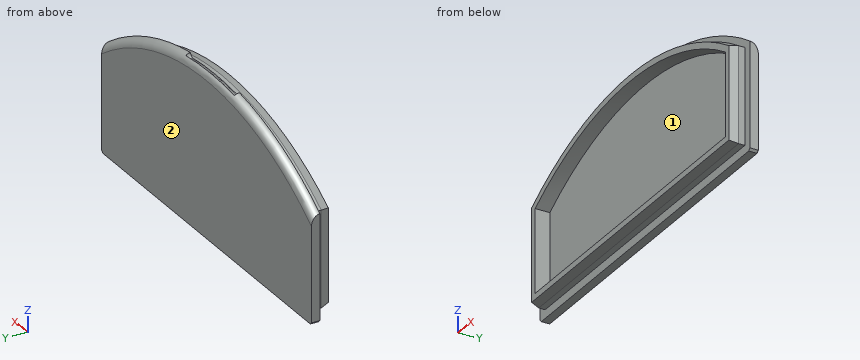
```python
from build123d import *
from OCP.BRepFilletAPI import BRepFilletAPI_MakeChamfer

# Parameters (mm, degrees)
EXTRUDE_1_DEPTH     = 4
CHAMFER_1_SIZE      = 1
EXTRUDE_2_DEPTH     = 7
CHAMFER_2_SIZE      = 4
CHAMFER_2_SIZE2     = 1.07179677
CUT_EXTRUDE_1_DEPTH = 2.5
FILLET_1_R          = 2
FILLET_2_R          = 4


with BuildPart() as part:
    # 스케치1 → 보스-돌출1 (new body)
    with BuildSketch(Plane(origin=(0, 0, 0), x_dir=(1, 0, 0), z_dir=(0, 1, 0))):
        with BuildLine():
            Line((85.8, -72), (85.8, -123.038042897))
            ThreePointArc((85.8, -123.038042897), (0, -150), (-85.8, -123.038042897))
            Line((-85.8, -123.038042897), (-85.8, -72))
            Line((-85.8, -72), (85.8, -72))
        make_face()
    extrude(amount=EXTRUDE_1_DEPTH)

    # 모따기1
    chamfer_1_edges = [part.edges().sort_by_distance(p)[0] for p in [
        (85.8, 2, 72),
        (-85.8, 2, 72),
    ]]
    chamfer(chamfer_1_edges, length=CHAMFER_1_SIZE)

    # 스케치2 → 보스-돌출2 (add)
    with BuildSketch(Plane.XZ):
        with BuildLine():
            Line((-81.7, 76.1), (-81.7, 121.964544028))
            ThreePointArc((-81.7, 121.964544028), (0, 146.8), (81.7, 121.964544028))
            Line((81.7, 121.964544028), (81.7, 76.1))
            Line((81.7, 76.1), (-81.7, 76.1))
        make_face()
        with BuildLine():
            Line((-77.8, 80), (-77.8, 119.745563592))
            ThreePointArc((-77.8, 119.745563592), (0, 142.8), (77.8, 119.745563592))
            Line((77.8, 119.745563592), (77.8, 80))
            Line((77.8, 80), (-77.8, 80))
        make_face(mode=Mode.SUBTRACT)
    extrude(amount=EXTRUDE_2_DEPTH)

    # 모따기2: one chamfer whose edges measure the first distance from different faces: ONE call of the kernel's chamfer builder (chamfer() names one face for all edges)
    chamfer_2_edges_1 = [part.edges().sort_by_distance(p)[0] for p in [
        (0, -7, 146.8),
    ]]
    chamfer_2_side_1 = [part.faces().sort_by_distance(p)[0] for p in [
        (0, -3.5, 146.8),
    ]]
    chamfer_2_edges_2 = [part.edges().sort_by_distance(p)[0] for p in [
        (-81.7, -7, 99.032272014),
    ]]
    chamfer_2_side_2 = [part.faces().sort_by_distance(p)[0] for p in [
        (-81.7, -3.5, 99.032272014),
    ]]
    chamfer_2_edges_3 = [part.edges().sort_by_distance(p)[0] for p in [
        (0, -7, 76.1),
    ]]
    chamfer_2_side_3 = [part.faces().sort_by_distance(p)[0] for p in [
        (0, -3.5, 76.1),
    ]]
    chamfer_2_edges_4 = [part.edges().sort_by_distance(p)[0] for p in [
        (81.7, -7, 99.032272014),
    ]]
    chamfer_2_side_4 = [part.faces().sort_by_distance(p)[0] for p in [
        (81.7, -3.5, 99.032272014),
    ]]
    chamfer_2 = BRepFilletAPI_MakeChamfer(part.part.solid().wrapped)
    for e in chamfer_2_edges_1:
        chamfer_2.Add(CHAMFER_2_SIZE, CHAMFER_2_SIZE2, e.wrapped, chamfer_2_side_1[0].wrapped)  # the first distance lies on this face
    for e in chamfer_2_edges_2:
        chamfer_2.Add(CHAMFER_2_SIZE, CHAMFER_2_SIZE2, e.wrapped, chamfer_2_side_2[0].wrapped)  # the first distance lies on this face
    for e in chamfer_2_edges_3:
        chamfer_2.Add(CHAMFER_2_SIZE, CHAMFER_2_SIZE2, e.wrapped, chamfer_2_side_3[0].wrapped)  # the first distance lies on this face
    for e in chamfer_2_edges_4:
        chamfer_2.Add(CHAMFER_2_SIZE, CHAMFER_2_SIZE2, e.wrapped, chamfer_2_side_4[0].wrapped)  # the first distance lies on this face
    add(Compound.cast(chamfer_2.Shape()), mode=Mode.REPLACE)

    # 스케치3 → 컷-돌출1 (cut)
    with BuildSketch(Plane.XZ):
        with BuildLine():
            Line((20, 146.642422239), (20, 148.660687473))
            ThreePointArc((20, 148.660687473), (0, 150), (-20, 148.660687473))
            Line((-20, 148.660687473), (-20, 146.642422239))
            ThreePointArc((-20, 146.642422239), (0, 148), (20, 146.642422239))
        make_face()
    extrude(amount=-CUT_EXTRUDE_1_DEPTH, mode=Mode.SUBTRACT)

    # 필렛1
    # the kernel refuses this fillet: 2 mm, written as the material it adds along each edge
    with BuildSketch(Plane(origin=(20, 0, 146.642422239), x_dir=(-0.991822496989378, 0, 0.12762497586975344), z_dir=(0, 1, 0))) as fillet_1_piece_1:
        with BuildLine():
            CenterArc((2.257580225, 1.999942607), FILLET_1_R, 179.947910746, 89.618025307)
            Line((0.257581052, 2.001760865), (0.217581068, 2.00179723))
            ThreePointArc((0.217581068, 2.00179723), (0.089117626, 1.005985431), (-0.0396729, 0.005104999))
            Line((-0.0396729, 0.005104999), (0.000303031, -0.039998852))
            ThreePointArc((0.000303031, -0.039998852), (1.12121434, -0.035752907), (2.242125649, -0.039998852))
            Line((2.242125649, -0.039998852), (2.24242868, 0))
        make_face()
    extrude(amount=2.5)
    with BuildSketch(Plane(origin=(-20, 0, 146.642422239), x_dir=(0, 0, 1), z_dir=(0, 1, 0))) as fillet_1_piece_2:
        with BuildLine():
            CenterArc((2.271711692, 1.983876229), FILLET_1_R, 173.101693725, 89.618025307)
            Line((0.286189906, 2.224091213), (0.24647947, 2.228895513))
            ThreePointArc((0.24647947, 2.228895513), (0.107634416, 1.11660857), (-0.039633087, 0.005405405))
            Line((-0.039633087, 0.005405405), (0, -0.04))
            ThreePointArc((0, -0.04), (1.009132617, -0.04), (2.013196305, -0.039677525))
            Line((2.013196305, -0.039677525), (2.018265235, 0))
        make_face()
    extrude(amount=2.5)
    with BuildSketch(Plane(origin=(0, 2.5, 0), x_dir=(-0.16852594692662803, 0, 0.9856972178171568), z_dir=(-0.9856972178171568, 0, -0.16852594692662803))) as fillet_1_piece_3:
        with BuildLine():
            CenterArc((148 + FILLET_1_R, -FILLET_1_R), FILLET_1_R, 90, 90)
            Line((148 + FILLET_1_R, 0), (148 + FILLET_1_R, FILLET_1_R * 0.02))
            Line((148 + FILLET_1_R, FILLET_1_R * 0.02), (148 - FILLET_1_R * 0.02, FILLET_1_R * 0.02))
            Line((148 - FILLET_1_R * 0.02, FILLET_1_R * 0.02), (148 - FILLET_1_R * 0.02, -FILLET_1_R))
            Line((148 - FILLET_1_R * 0.02, -FILLET_1_R), (148, -FILLET_1_R))
        make_face()
    revolve(axis=Axis((0, 2.5, 0), (0, 1, 0)), revolution_arc=19.4042511)

    # 필렛2
    # the kernel refuses this fillet: 4 mm, written as the material it takes off along each edge
    with BuildSketch(Plane(origin=(0, 4, 0), x_dir=(0.6253849976440692, 0, 0.7803163491313813), z_dir=(0.7803163491313813, 0, -0.6253849976440692))) as fillet_2_piece_1_section:
        with BuildLine():
            CenterArc((150 - FILLET_2_R, FILLET_2_R), FILLET_2_R, 270, 90)
            Line((150 - FILLET_2_R, 0), (150 - FILLET_2_R, -FILLET_2_R * 0.02))
            Line((150 - FILLET_2_R, -FILLET_2_R * 0.02), (150 + FILLET_2_R * 0.02, -FILLET_2_R * 0.02))
            Line((150 + FILLET_2_R * 0.02, -FILLET_2_R * 0.02), (150 + FILLET_2_R * 0.02, FILLET_2_R))
            Line((150 + FILLET_2_R * 0.02, FILLET_2_R), (150, FILLET_2_R))
        make_face()
    fillet_2_piece_1 = revolve(axis=Axis((0, 4, 0), (0, -1, 0)), revolution_arc=77.420901677, mode=Mode.PRIVATE)
    fillet_2_piece_1 = split(fillet_2_piece_1, bisect_by=Plane(origin=(85.8, 2.892558324, 148.892558324), z_dir=(-1, 0, 0)), keep=Keep.TOP, mode=Mode.PRIVATE)
    fillet_2_piece_1 = split(fillet_2_piece_1, bisect_by=Plane(origin=(-85.8, 2.892558324, 148.892558324), z_dir=(1, 0, 0)), keep=Keep.TOP, mode=Mode.PRIVATE)
    add(fillet_2_piece_1, mode=Mode.SUBTRACT)


solid = part.part
```
Verification items for the finished model (mm, model axes). Face numbers are marked on the shaded views. Coordinates: 2 decimals unless noted, no trailing zeros. Order: outer loops, then holes, each group sorted by start corner. A loop starts at its lowest first (then second) coordinate and runs counter-clockwise, first axis right, second up. Notation, with made-up numbers: (42, 65.5) -> (51, 65.5) arc R25 cw to (51, 87.5) -> close; hole circle Ø9 at (12.25, -3). An arc over 180 degrees is marked (long way). Put each result on its own line as item: value. Start each with the question number.
1) Release check for a two-part mould opening along Z. For the marked faces 1 and 2 record: pulls with the +Z half, pulls with the -Z half, needs draft (parallel to the pull), parting line crosses it, or undercut.
2) Material ranges on L1, parallel to X at y = -1, z = 106.5; L2, parallel to Y at x = 12, z = 81.5; L3, parallel to Z at x = -37, y = -4.25, recorded low to high.
3) Cross-section at A-A (z = 106). Enter the section's corners in (x, y), plus the area to 3 significant figures.
4) Go/stop test with flat-tipped pins: pin 1 (2.5 mm diameter, centred on y = -2, z = 88.5, fed in from -X); pin 2 (1 mm diameter, centred on y = -3, z = 129.5, fed in from +X); pin 3 (3.5 mm diameter, centred on x = 11, y = -4, fed in from +Z). Record where each tip stops, or that it passes through.
Geometry check:
1. face 1: undercut
1. face 2: needs draft
2. L1: x = -81.7 to -77.8, 77.8 to 81.7
2. L2: y = 0 to 4
2. L3: z = 76.43 to 80, 137.92 to 141.71
3. outline: (-85.8, 0) -> (-81.7, 0) -> (-81.7, -3) -> (-80.63, -7) -> (-77.8, -7) -> (-77.8, 0) -> (77.8, 0) -> (77.8, -7) -> (80.63, -7) -> (81.7, -3) -> (81.7, 0) -> (85.8, 0) -> (85.8, 4) -> (-85.8, 4) -> close
3. area: 737 mm^2
4. pin 1: stops at x = -81.7
4. pin 2: stops at x = 70.07
4. pin 3: stops at z = 146.49
